Can you work these out from the model? Positions are in its coordinate system, mm. A direction names the side the tool comes from. Coordinates: 2 decimals unless noted, no trailing zeros. Order: outer loops, then holes, each group sorted by start corner. A loop starts at its lowest first (then second) coordinate and runs counter-clockwise, first axis right, second up. Notation, with made-up numbers: (-16.75, -30.5) -> (40.25, -30.5) arc R28 ccw to (40.25, 7.5) -> close; hole circle Ø3 at (7, 39.5). An arc over 180 degrees is marked (long way). Answer in a Markdown table with one row per item.
```python
from build123d import *

# Parameters (mm, degrees)
F0_R     = 12.5
F1_DEPTH = 12


with BuildPart() as f1:
    # F0 (on Right) → F1 (new body)
    with BuildSketch(Plane.YZ):
        with BuildLine():
            ThreePointArc((-37.205878, 454.6875), (-2.348359, 412.573603), (37.5, 450))
            ThreePointArc((37.5, 450), (37.426397, 452.348359), (37.205878, 454.6875))
            ThreePointArc((37.205878, 454.6875), (0, 487.5), (-37.205878, 454.6875))
        make_face()
        with Locations((0, 450)):
            Circle(F0_R, mode=Mode.SUBTRACT)
        with BuildLine():
            ThreePointArc((37.205878, 454.6875), (37.426397, 452.348359), (37.5, 450))
            ThreePointArc((37.5, 450), (-2.348359, 412.573603), (-37.205878, 454.6875))
            Line((-37.205878, 454.6875), (-62.009796, 257.8125))
            ThreePointArc((-62.009796, 257.8125), (0, 312.5), (62.009796, 257.8125))
            Line((62.009796, 257.8125), (37.205878, 454.6875))
        make_face()
        with Locations((-12.5, 393.8)):
            Circle(F0_R, mode=Mode.SUBTRACT)
        with BuildLine():
            ThreePointArc((62.5, 250), (62.377329, 253.913932), (62.009796, 257.8125))
            ThreePointArc((62.009796, 257.8125), (0, 312.5), (-62.009796, 257.8125))
            ThreePointArc((-62.009796, 257.8125), (-62.495054, 250.786242), (-62.186715, 243.75))
            ThreePointArc((-62.186715, 243.75), (0, 187.5), (62.186715, 243.75))
            ThreePointArc((62.186715, 243.75), (62.42163, 246.871077), (62.5, 250))
        make_face()
        with Locations((0, 250)):
            Circle(F0_R, mode=Mode.SUBTRACT)
        with BuildLine():
            ThreePointArc((62.186715, 243.75), (0, 187.5), (-62.186715, 243.75))
            Line((-62.186715, 243.75), (-37.312029, -3.75))
            ThreePointArc((-37.312029, -3.75), (-1.877354, 37.452978), (37.5, 0))
            ThreePointArc((37.5, 0), (26.985859, -26.03869), (1.339286, -37.476077))
            Line((1.339286, -37.476077), (176.116071, -31.230064))
            ThreePointArc((176.116071, -31.230064), (143.75, 0), (176.116071, 31.230064))
            Line((176.116071, 31.230064), (74.675591, 34.855251))
            ThreePointArc((74.675591, 34.855251), (52.209448, 45.556532), (44.650341, 69.265283))
            Line((44.650341, 69.265283), (62.186715, 243.75))
        make_face()
        with BuildLine():
            ThreePointArc((37.5, 0), (-1.877354, 37.452978), (-37.312029, -3.75))
            ThreePointArc((-37.312029, -3.75), (-24.655053, -28.25559), (1.339286, -37.476077))
            ThreePointArc((1.339286, -37.476077), (26.985859, -26.03869), (37.5, 0))
        make_face()
        Circle(F0_R, mode=Mode.SUBTRACT)
        with BuildLine():
            ThreePointArc((176.116071, 31.230064), (143.75, 0), (176.116071, -31.230064))
            ThreePointArc((176.116071, -31.230064), (197.488216, -21.698909), (206.25, 0))
            ThreePointArc((206.25, 0), (197.488216, 21.698909), (176.116071, 31.230064))
        make_face()
        with Locations((175, 0)):
            Circle(F0_R, mode=Mode.SUBTRACT)
    extrude(amount=F1_DEPTH)


solid = f1.part
```
(1) Suppose I cut it at B-B (x = 5). Please give me the cut outline in (y, z).
Response values:
| item | result |
|---|---|
| outline | (-62.19, 243.75) -> (-37.31, -3.75) arc R37.5 ccw to (1.34, -37.48) -> (176.12, -31.23) arc R31.25 ccw to (176.12, 31.23) -> (74.68, 34.86) arc R31.3 cw to (44.65, 69.27) -> (62.19, 243.75) arc R62.5 ccw to (62.5, 250) arc R62.5 ccw to (62.01, 257.81) -> (37.21, 454.69) arc R37.5 ccw to (-37.21, 454.69) -> (-62.01, 257.81) arc R62.5 ccw to start; hole circle Ø25 at (-12.5, 393.8); hole circle Ø25 at (0, 0); hole circle Ø25 at (0, 250); hole circle Ø25 at (0, 450); hole circle Ø25 at (175, 0) |
(2) Suppose I cut it at C-C (z = 92.5). Please give me the cut outline in (x, y), and give its area (3 significant figures).
Response values:
| item | result |
|---|---|
| outline | (0, -46.99) -> (12, -46.99) -> (12, 46.99) -> (0, 46.99) -> close |
| area | 1,130 mm2 |
(3) Will these pins go through, and if not, where does the flat tip stop? pin 1 Ø20 at (y, z) = (175, 0) entering from +X; pin 2 Ø4 at (x, z) = (8.5, 373.5) entering from -Y; pin 3 Ø4 at (x, z) = (2.5, 22.5) entering from -Y; pin 4 Ø2 at (x, z) = (1.5, 90) entering from +Y.
Response values:
| item | result |
|---|---|
| pin 1 | through |
| pin 2 | y = -47.69 |
| pin 3 | y = -40.15 |
| pin 4 | y = 46.83 |
(4) Suppose I cut it at A-A (z = 393.8). Please give me the cut outline in (x, y), and give its area (3 significant figures).
Response values:
| item | result |
|---|---|
| outline | (0, -44.88) -> (12, -44.88) -> (12, -25) -> (0, -25) -> close; (0, 0) -> (12, 0) -> (12, 44.88) -> (0, 44.88) -> close |
| area | 777 mm2 |
(5) I need wall thicknesses on line 1 (Z direction, x = 2.5, y = 175); line 2 (Z direction, x = 1, y = 173.5); line 3 (Y direction, x = 8.75, z = -7.5). Which ranges of each line are inside material? Lowest first, please. Write a range as [from, to].
Response values:
| item | result |
|---|---|
| line 1 | [-31.27, -12.5], [12.5, 31.27] |
| line 2 | [-31.32, -12.41], [12.41, 31.32] |
| line 3 | [-36.74, -10], [10, 165], [185, 205.34] |
(6) We'd pull the mould along Y, two halves only. Please class faces 3 (the flat face through (12, 10, 170)), 4 (the cylindrical face through (5.916, 186.923, 3.755)), 5 (the flat face through (5.92, 49.78, 354.87)): +Y half, -Y half, draft (parallel to the pull), parting line (faces both ways), or undercut.
Response values:
| item | result |
|---|---|
| face 3 | draft |
| face 4 | undercut |
| face 5 | +Y half |
(7) On a 3-axis mill with a long thin cutter (end or side, diameter ignored), from which of +Z, -Z, +X, -X, +Y, -Y can I reach the whole of each face in a straight line? I mean faces 1 (the flat face through (5.916, 53.296, 155.286)), 2 (the cylindrical face through (5.92, 5.77, 438.91)). Say none if no direction works.
Response values:
| item | result |
|---|---|
| face 1 | +X, -X, +Y |
| face 2 | +X, -X |
